Autodesk Inventor part; units mm, degrees
ref_plane "YZ Plane" through (0, 0, 0) normal (1, 0, 0) x (0, 1, 0)
ref_plane "XZ Plane" through (0, 0, 0) normal (0, 1, 0) x (-1, 0, 0)
ref_plane "XY Plane" through (0, 0, 0) normal (0, 0, 1) x (1, 0, 0)
sketch "Skizze1" plane through (0, 0, 0) normal (0, 1, 0) x (-1, 0, 0)
  line L0 (1.5, 0) -> (-1.5, 0)
  line L1 (1.5, 1.5) -> (-1.5, 1.5)
  line L2 (-1.5, 1.5) -> (-1.5, 2)
  line L3 (-1.5, 2) -> (-1.3, 2)
  line L4 (-1.3, 2) -> (-1.3, 3)
  line L5 (-1.3, 3) -> (-1.5, 3)
  line L6 (-1.5, 3) -> (-1.5, 3.5)
  line L7 (-1.5, 3.5) -> (1.5, 3.5)
  line L8 (1.5, 3.5) -> (1.5, 3)
  line L9 (1.5, 3) -> (1.3, 3)
  line L10 (1.3, 3) -> (1.3, 2)
  line L11 (1.3, 2) -> (1.5, 2)
  line L12 (1.5, 1.5) -> (1.5, 2)
  line L13 (0, -0.7) -> (0, 4.2)
  point P0 (0, 0)
  dimension "d0" = 3
  dimension "d1" = 7
  dimension "d2" = 3
  dimension "d3" = 0.2
  dimension "d4" = 0.5
  dimension "d5" = 0.5
revolve "Umdrehung1" add sketch "Skizze1" angle 360 about axis through (-1.5, 0, 0) along (1, 0, 0)
properties part number "Kugellager 683-ZZ" material "Stahl, weich, geschweißt"
Here's how the part is built. I have some questions about the finished solid (model axes, mm). Give positions to 0.01 mm unless a question says otherwise; leave off trailing zeros. Loops run counter-clockwise (first coordinate to the right, second up) from the corner with the lowest first, then second, coordinate; pieces in that order, holes last. Notation, with made-up numbers: M 55.25,-25 L 60.25,-25 A22 cw 60.25,-13 Z; hole C 85,79 d2. An arc over 180 degrees is marked long. Return JSON: item names as keys, results as strings.
Item 1: Imagine slicing it at D-D on z = -2.5. List the corners of the cut face in (x, y) for me.
A:
{"outline": "M -1.5,-2.45 L 1.5,-2.45 L 1.5,-1.66 L 1.3,-1.66 L 1.3,1.66 L 1.5,1.66 L 1.5,2.45 L -1.5,2.45 L -1.5,1.66 L -1.3,1.66 L -1.3,-1.66 L -1.5,-1.66 Z"}
Item 2: Imagine slicing it at A-A on z = 0. List the corners of the cut face in (x, y) for me.
A:
{"outline": "M -1.5,-3.5 L 1.5,-3.5 L 1.5,-3 L 1.3,-3 L 1.3,-2 L 1.5,-2 L 1.5,-1.5 L -1.5,-1.5 L -1.5,-2 L -1.3,-2 L -1.3,-3 L -1.5,-3 Z; M -1.5,1.5 L 1.5,1.5 L 1.5,2 L 1.3,2 L 1.3,3 L 1.5,3 L 1.5,3.5 L -1.5,3.5 L -1.5,3 L -1.3,3 L -1.3,2 L -1.5,2 Z"}
Item 3: Please list where these lines run through material, in increasing order: line 1 (Y direction, x = -1.4, z = 0); line 2 (Z direction, x = -0.6, y = 0).
A:
{"line 1": "y = -3.5 to -3, -2 to -1.5, 1.5 to 2, 3 to 3.5", "line 2": "z = -3.5 to -1.5, 1.5 to 3.5"}
Item 4: Imagine slicing it at C-C on x = -1.05. List the corners of the cut face in (y, z) for me.
A:
{"outline": "C 0,0 d7; hole C 0,0 d3"}
Item 5: I'm going to push a flat-ended pin straight in: pin 1 Ø1 at (x, z) = (0, -2.5) entering from +Y. Where does the tip first touch, or does it pass through?
A:
{"pin 1": "stops at y = 2.87"}
Item 6: Thinking about a two-plate mould opening in Z: for faces 1 (the flat face through (1.3, 2, 1)), 2 (the cylindrical face through (-0.021, -1.341, 3.233)), 3 (the flat face through (-1.3, 2, 1)), 4 (the flat face through (-1.5, -1, 3)), which applies, released by +Z, released by -Z, zero draft, split by the parting line, or undercut?
A:
{"face 1": "undercut", "face 2": "split by the parting line", "face 3": "undercut", "face 4": "zero draft"}
